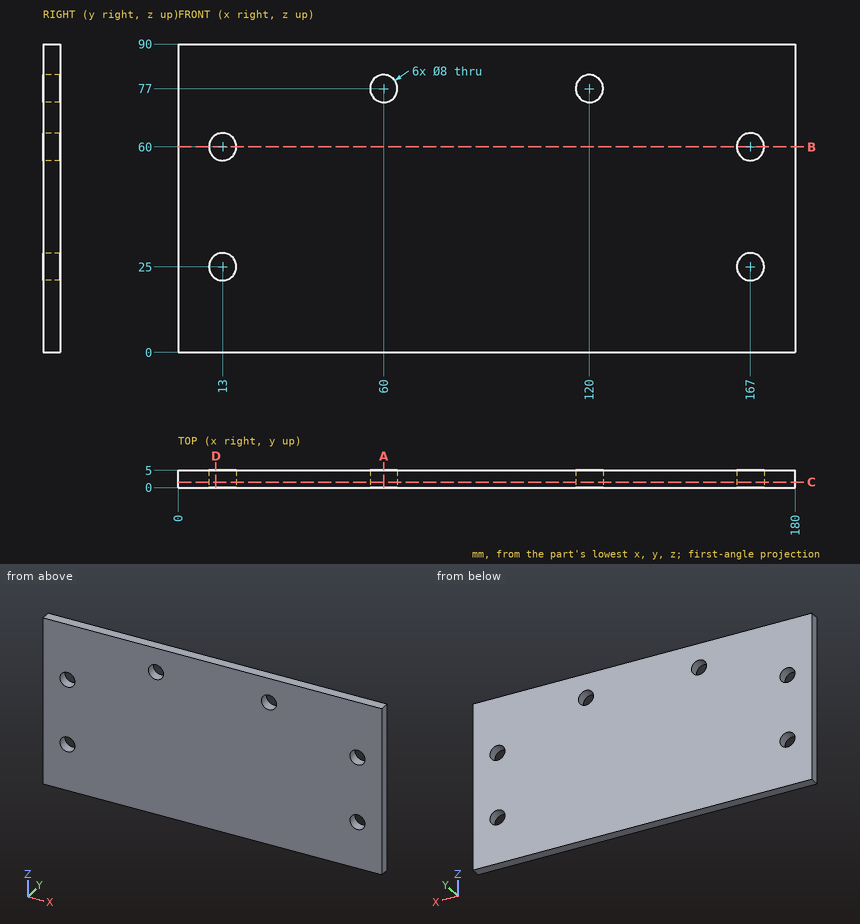
Geometry check sheet. Reference: drawing and pictorial views, mm from the part's lowest x, y, z. Coordinates: 2 decimals unless noted, no trailing zeros. Order: outer loops, then holes, each group sorted by start corner. A loop starts at its lowest first (then second) coordinate and runs counter-clockwise, first axis right, second up. Notation, with made-up numbers: (-8.5, -12.75) - (12.5, -12.75) arc R17 ccw to (12.5, 3.25) - close; hole circle Ø1 at (59, -34). An arc over 180 degrees is marked (long way). One line per item, written item: value.
(1) Sectioned sample at A-A (x = 60). Enter the section's corners in (y, z).
Data:
outline: (0, 0) - (5, 0) - (5, 73) - (0, 73) - close; (0, 81) - (5, 81) - (5, 90) - (0, 90) - close
(2) Depth check by flat-ended pin: pin 1 Ø5 at (x, z) = (60, 77) entering from -Y; pin 2 Ø2 at (x, y) = (132.5, 3) entering from -Z. Enter the tip coordinate at first touch or a pass-through.
Data:
pin 1: passes through
pin 2: stops at z = 0
(3) Sectioned sample at B-B (z = 60). Enter the section's corners in (x, y), and give its area (3 significant figures).
Data:
outline: (0, 0) - (9, 0) - (9, 5) - (0, 5) - close; (17, 0) - (163, 0) - (163, 5) - (17, 5) - close; (171, 0) - (180, 0) - (180, 5) - (171, 5) - close
area: 820 mm^2
(4) Thickness scan on probe 1 along X at (y, z) = (1.6, 60); probe 2 along Z at (x, y) = (169.5, 0.7); probe 3 along Z at (x, y) = (12, 3.8). Record the ranges inside material, lowest first. Write a range as from..to.
Data:
probe 1: x = 0..9, 17..163, 171..180
probe 2: z = 0..21.88, 28.12..56.88, 63.12..90
probe 3: z = 0..21.13, 28.87..56.13, 63.87..90
(5) Sectioned sample at D-D (x = 11). Enter the section's corners in (y, z), and give its area (3 significant figures).
Data:
outline: (0, 0) - (5, 0) - (5, 21.54) - (0, 21.54) - close; (0, 28.46) - (5, 28.46) - (5, 56.54) - (0, 56.54) - close; (0, 63.46) - (5, 63.46) - (5, 90) - (0, 90) - close
area: 381 mm^2
(6) Sectioned sample at C-C (y = 1.6). Enter the section's corners in (x, z), and give its area (3 significant figures).
Data:
outline: (0, 0) - (180, 0) - (180, 90) - (0, 90) - close; hole circle Ø8 at (13, 25); hole circle Ø8 at (13, 60); hole circle Ø8 at (60, 77); hole circle Ø8 at (120, 77); hole circle Ø8 at (167, 25); hole circle Ø8 at (167, 60)
area: 15,900 mm^2
